Autodesk Inventor part; units mm, degrees
ref_plane "YZ Plane" through (0, 0, 0) normal (1, 0, 0) x (0, 1, 0)
ref_plane "XZ Plane" through (0, 0, 0) normal (0, 1, 0) x (-1, 0, 0)
ref_plane "XY Plane" through (0, 0, 0) normal (0, 0, 1) x (1, 0, 0)
sketch "Boceto1" plane through (0, 0, 0) normal (0, 1, 0) x (-1, 0, 0)
  line L0 (1.7076, 3.014) -> (3.464, 0.0282)
  line L1 (3.464, 0.0282) -> (1.7564, -2.9858)
  line L2 (1.7564, -2.9858) -> (-1.7076, -3.014)
  line L3 (-1.7076, -3.014) -> (-3.464, -0.0282)
  line L4 (-3.464, -0.0282) -> (-1.7564, 2.9858)
  line L5 (-1.7564, 2.9858) -> (1.7076, 3.014)
  point P0 (0, 0)
  point P1 (0, 0)
  dimension "d0" = 6
extrude "Extrusión1" add sketch "Boceto1" along normal blind 19.1
sketch "Boceto2" plane through (0, 19.1, 0) normal (0, 1, 0) x (1, 0, 0)
  point P0 (0, 0)
  point P1 (0, 0)
hole "Agujero1" at (0, 19.1, 0) direction (0, -1, 0) diameter 2.459 end through all
properties part number "pataUnion" material "Poliestireno"
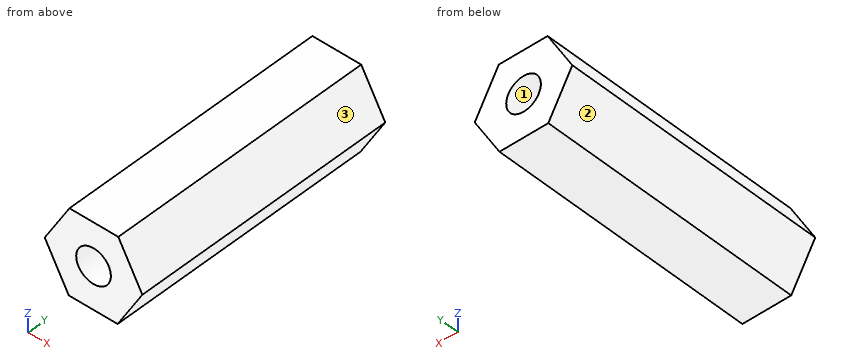
Geometry: final body of the model. Coordinates: model frame, mm. Face numbers are marked on the shaded views. Round coordinates to 2 decimals unless told otherwise and drop trailing zeros. Loops run counter-clockwise (first coordinate to the right, second up) from the corner with the lowest first, then second, coordinate; pieces in that order, holes last. Notation, with made-up numbers: (60.25, 3) - (88.25, 3) arc R14 ccw to (88.25, 12) - close; hole circle Ø7 at (77.5, -26). An arc over 180 degrees is marked (long way). Write each question's results on one line, items separated by ' | '. Start each with the question number.
1) Cut plane D-D on z = -1.75. Return loops of the section in (x, y), then the cut area to 3 significant figures.
2) Cut plane B-B on x = 0. Return loops of the section in (y, z), then the cut area to 3 significant figures.
3) First-contact query: P1, Ø1.5, axis at y = 9, z = -1.5, coming from the -X side; P2, Ø3, axis at y = 8, z = 2.5, coming from the -X side; P3, Ø2, axis at x = 0, z = 0, coming from the +Y side; P4, Ø3, axis at x = -1.5, y = 9.5, coming from the -Z side. Flat tips, straight axial feed; report the tip coordinate or a pass-through.
4) Cut plane A-A on y = 5. Return loops of the section in (x, z), then the cut area to 3 significant figures.
5) Mould query, pull axis Z, two halves, no side actions, for the marked faces 1, 2 and 3. Classes: released by +Z, released by -Z, zero draft, split by the parting line, or undercut.
6) Line query: probe 1 along X at (y, z) = (4.75, 0); probe 2 along Z at (x, y) = (0, 8.5); probe 3 along Z at (x, y) = (0.5, 8). Output: solid intervals per line, ascending. Write a range as [from, to].
7) Cut plane C-C on z = -1. Return loops of the section in (x, y), then the cut area to 3 significant figures.
Verdict:
1) outline: (-2.46, 0) - (2.45, 0) - (2.45, 19.1) - (-2.46, 19.1) - close | area: 93.7 mm2
2) outline: (0, -3) - (19.1, -3) - (19.1, -1.23) - (0, -1.23) - close; (0, 1.23) - (19.1, 1.23) - (19.1, 3) - (0, 3) - close | area: 67.6 mm2
3) P1: stops at x = -3.02 | P2: stops at x = -2.89 | P3: passes through | P4: stops at z = -3
4) outline: (-3.46, 0.03) - (-1.76, -2.99) - (1.71, -3.01) - (3.46, -0.03) - (1.76, 2.99) - (-1.71, 3.01) - close; hole circle Ø2.46 at (0, 0) | area: 26.4 mm2
5) face 1: undercut | face 2: released by -Z | face 3: released by +Z
6) probe 1: x = [-3.45, -1.23], [1.23, 3.45] | probe 2: z = [-3, -1.23], [1.23, 3] | probe 3: z = [-3, -1.12], [1.12, 3]
7) outline: (-2.88, 0) - (-0.72, 0) - (-0.72, 19.1) - (-2.88, 19.1) - close; (0.72, 0) - (2.89, 0) - (2.89, 19.1) - (0.72, 19.1) - close | area: 83.0 mm2
